```python
from build123d import *

# Parameters (mm, degrees)
SKETCH1_W               = 25.4
SKETCH1_H               = 50.8
SKETCH1_W_2             = 20.32
SKETCH1_H_2             = 45.72
BOSS_EXTRUDE1_DEPTH     = 114.3
SKETCH6_W               = 25.4
SKETCH6_H               = 50.8
SKETCH6_W_2             = 20.32
SKETCH6_H_2             = 45.72
BOSS_EXTRUDE4_DEPTH     = 38.1
SKETCH2_R               = 2.032
CUT_EXTRUDE1_DEPTH      = 162.144934764
CUT_EXTRUDE2_DEPTH      = 157.576115675
CUT_EXTRUDE2_DEPTH_BACK = 157.576115675
SKETCH3_R               = 2.032
SKETCH7_W               = 25.4
SKETCH7_H               = 50.8
CUT_EXTRUDE3_DEPTH      = 12.7
SKETCH8_R               = 3.302
CUT_EXTRUDE5_DEPTH      = 157.576115675
SKETCH9_R               = 2.032
CUT_EXTRUDE6_DEPTH      = 157.576115675


with BuildPart() as part:
    # Sketch1 → Boss-Extrude1 (new body)
    with BuildSketch(Plane.XY):
        Rectangle(SKETCH1_W, SKETCH1_H)
        Rectangle(SKETCH1_W_2, SKETCH1_H_2, mode=Mode.SUBTRACT)
    extrude(amount=BOSS_EXTRUDE1_DEPTH)

    # Sketch6 → Boss-Extrude4 (add)
    with BuildSketch(Plane.XY.offset(114.3)):
        Rectangle(SKETCH6_W, SKETCH6_H)
        Rectangle(SKETCH6_W_2, SKETCH6_H_2, mode=Mode.SUBTRACT)
    extrude(amount=BOSS_EXTRUDE4_DEPTH)

    # Sketch2 → Cut-Extrude1 (cut, through all)
    with BuildSketch(Plane(origin=(0, 25.4, 0), x_dir=(1, 0, 0), z_dir=(0, 1, 0))):
        Circle(SKETCH2_R)
        with Locations(Location((0, -12.7, 0), (0, 0, 270))):
            Circle(SKETCH2_R)
        with Locations(Location((0, -25.4, 0), (0, 0, 270))):
            Circle(SKETCH2_R)
        with Locations(Location((0, -38.1, 0), (0, 0, 270))):
            Circle(SKETCH2_R)
        with Locations(Location((0, -50.8, 0), (0, 0, 270))):
            Circle(SKETCH2_R)
        with Locations(Location((0, -63.5, 0), (0, 0, 270))):
            Circle(SKETCH2_R)
        with Locations(Location((0, -76.2, 0), (0, 0, 270))):
            Circle(SKETCH2_R)
        with Locations(Location((0, -88.9, 0), (0, 0, 270))):
            Circle(SKETCH2_R)
        with Locations(Location((0, -101.6, 0), (0, 0, 270))):
            Circle(SKETCH2_R)
        with Locations(Location((0, -114.3, 0), (0, 0, 270))):
            Circle(SKETCH2_R)
        with Locations(Location((0, -127, 0), (0, 0, 270))):
            Circle(SKETCH2_R)
        with Locations(Location((0, -139.7, 0), (0, 0, 270))):
            Circle(SKETCH2_R)
        with Locations((0, -152.4)):
            Circle(SKETCH2_R)
        with Locations((0, -165.1)):
            Circle(SKETCH2_R)
        with Locations((0, -177.8)):
            Circle(SKETCH2_R)
        with Locations((0, -190.5)):
            Circle(SKETCH2_R)
        with Locations((0, -203.2)):
            Circle(SKETCH2_R)
        with Locations((0, -215.9)):
            Circle(SKETCH2_R)
        with Locations((0, -228.6)):
            Circle(SKETCH2_R)
        with Locations((0, -241.3)):
            Circle(SKETCH2_R)
    extrude(amount=-CUT_EXTRUDE1_DEPTH, mode=Mode.SUBTRACT)

    # Sketch3 → Cut-Extrude2 (cut, two sides: drawn at the far end of the back side and taken through both)
    with BuildSketch(Plane.ZY.offset(12.7).offset(-CUT_EXTRUDE2_DEPTH_BACK)):
        with Locations((101.6, 12.7)):
            Circle(SKETCH3_R)
        with Locations((101.6, 0)):
            Circle(SKETCH3_R)
        with Locations((101.6, -12.7)):
            Circle(SKETCH3_R)
        with Locations((88.9, 0)):
            Circle(SKETCH3_R)
        with Locations((88.9, -12.7)):
            Circle(SKETCH3_R)
        with Locations((76.2, 0)):
            Circle(SKETCH3_R)
        with Locations((76.2, -12.7)):
            Circle(SKETCH3_R)
        with Locations((88.9, 12.7)):
            Circle(SKETCH3_R)
        with Locations((76.2, 12.7)):
            Circle(SKETCH3_R)
    extrude(amount=CUT_EXTRUDE2_DEPTH + CUT_EXTRUDE2_DEPTH_BACK, mode=Mode.SUBTRACT)

    # Sketch7 → Cut-Extrude3 (cut)
    with BuildSketch(Plane(origin=(0, 0, 0), x_dir=(-1, 0, 0), z_dir=(0, 0, -1))):
        Rectangle(SKETCH7_W, SKETCH7_H)
    extrude(amount=-CUT_EXTRUDE3_DEPTH, mode=Mode.SUBTRACT)

    # Sketch8 → Cut-Extrude5 (cut, through all)
    with BuildSketch(Plane.ZY.offset(12.7)):
        with Locations((25.4, 12.7)):
            Circle(SKETCH8_R)
        with Locations((25.4, -12.7)):
            Circle(SKETCH8_R)
        with Locations((50.8, -12.7)):
            Circle(SKETCH8_R)
        with Locations((50.8, 12.7)):
            Circle(SKETCH8_R)
    extrude(amount=-CUT_EXTRUDE5_DEPTH, mode=Mode.SUBTRACT)

    # Sketch9 → Cut-Extrude6 (cut, through all)
    with BuildSketch(Plane.ZY.offset(12.7)):
        with Locations((146.05, 12.7)):
            Circle(SKETCH9_R)
        with Locations((146.05, 0)):
            Circle(SKETCH9_R)
        with Locations((146.05, -12.7)):
            Circle(SKETCH9_R)
        with Locations((133.35, 0)):
            Circle(SKETCH9_R)
        with Locations((133.35, -12.7)):
            Circle(SKETCH9_R)
        with Locations((120.65, 0)):
            Circle(SKETCH9_R)
        with Locations((120.65, -12.7)):
            Circle(SKETCH9_R)
        with Locations((133.35, 12.7)):
            Circle(SKETCH9_R)
        with Locations((120.65, 12.7)):
            Circle(SKETCH9_R)
    extrude(amount=-CUT_EXTRUDE6_DEPTH, mode=Mode.SUBTRACT)


solid = part.part
```
Geometry: final body of the model. Coordinates: model frame, mm. A direction names the side the tool comes from. Coordinates: 2 decimals unless noted, no trailing zeros. Order: outer loops, then holes, each group sorted by start corner. A loop starts at its lowest first (then second) coordinate and runs counter-clockwise, first axis right, second up. Notation, with made-up numbers: (54, 6.25) - (90, 6.25) arc R11 cw to (90, 18.25) - close; hole circle Ø2 at (-33.75, -28). An arc over 180 degrees is marked (long way). Write each question's results on one line, items separated by ' | '.
1) Section C-C, the plane y = 3.5. Return loops of the section in (x, z), plus the area to 3 significant figures.
Results list:
outline: (-12.7, 12.7) - (-10.16, 12.7) - (-10.16, 152.4) - (-12.7, 152.4) - close; (10.16, 12.7) - (12.7, 12.7) - (12.7, 152.4) - (10.16, 152.4) - close | area: 710 mm^2
2) Set-up query: faces 3 (the cylindrical face through (11.45, 12.79, 74.17)), 4 (the flat face through (-10.16, 0, 82)). Return all of +Z, -Z, +X, -X, +Y, -Y with unobstructed straight access to the full face (end or side cutting, diameter ignored); none if empty.
Results list:
face 3: +X, -X | face 4: +Z, -Z
3) Section A-A, the plane x = -3.25. Return loops of the section in (y, z).
Results list:
outline: (-25.4, 12.7) - (-22.86, 12.7) - (-22.86, 152.4) - (-25.4, 152.4) - close; (22.86, 12.7) - (25.4, 12.7) - (25.4, 152.4) - (22.86, 152.4) - close
4) Line query: line 1 (Y direction, x = -11.1, z = 133.35); line 2 (Y direction, x = -11.95, z = 25.4); line 3 (Y direction, x = -8, z = 116). Output: solid intervals per line, ascending. Write a range as from..to.
Results list:
line 1: -25.4..-14.73, -10.67..-2.03, 2.03..10.67, 14.73..25.4 | line 2: -25.4..-16, -9.4..9.4, 16..25.4 | line 3: -25.4..-22.86, 22.86..25.4
5) Pull-direction query (Y, two-part tool) for faces 1 (the flat face through (12.7, 0, 82)), 2 (the flat face through (0, -22.86, 82)); classes: pulls with the +Y half, pulls with the -Y half, needs draft (parallel to the pull), parting line crosses it, or undercut.
Results list:
face 1: needs draft | face 2: undercut
6) Section D-D, the plane z = 98. Return loops of the section in (x, y), plus the area to 3 significant figures.
Results list:
outline: (-12.7, -25.4) - (12.7, -25.4) - (12.7, 25.4) - (-12.7, 25.4) - close; hole (-10.16, -22.86) - (10.16, -22.86) - (10.16, 22.86) - (-10.16, 22.86) - close | area: 361 mm^2
7) Section B-B, the plane z = 50.8. State how many separate pieces and enclosed holes the cut face has, plus the area to 3 significant figures.
Results list:
separate pieces: 6 | enclosed holes: 0 | area: 274 mm^2
